The model under review builds one solid part; all positions refer to its coordinate system, in mm. A direction names the side the tool comes from. Coordinates: 2 decimals unless noted, no trailing zeros. Loops run counter-clockwise (first coordinate to the right, second up) from the corner with the lowest first, then second, coordinate; pieces in that order, holes last. Notation, with made-up numbers: (-20.75, 88.25) -> (12.25, 88.25) arc R21 cw to (12.25, 112.25) -> close; hole circle Ø6 at (23, 41.25). An arc over 180 degrees is marked (long way). One line per question, with ' | ' between items. Start each with the question number.
from build123d import *

# Parameters (mm, degrees)
F0_R     = 3
F1_DEPTH = 3.5
F2_W     = 14
F2_H     = 12.5
F3_DEPTH = 0.7
F4_R     = 10
F4_R_2   = 8.4
F5_DEPTH = 20
F6_R     = 10
F6_R_2   = 5
F7_DEPTH = 2


with BuildPart() as f1:
    # F0 (on Top) → F1 (new body)
    with BuildSketch(Plane.XY):
        with BuildLine():
            Line((-7, 37.141428), (-7, 7.141428))
            ThreePointArc((-7, 7.141428), (0, -10), (7, 7.141428))
            Line((7, 7.141428), (7, 37.141428))
            Line((7, 37.141428), (1.936133, 37.141428))
            Line((1.936133, 37.141428), (1.936133, 9.810779))
            ThreePointArc((1.936133, 9.810779), (-0.065184, 9.999788), (-2.063867, 9.784705))
            Line((-2.063867, 9.784705), (-2.063867, 37.141428))
            Line((-2.063867, 37.141428), (-7, 37.141428))
        make_face()
        Circle(F0_R, mode=Mode.SUBTRACT)
    extrude(amount=F1_DEPTH)

    # F2 (on face) → F3 (cut)
    with BuildSketch(Plane.XY.offset(3.5)):
        with Locations((0, 30.891428)):
            Rectangle(F2_W, F2_H)
    extrude(amount=-F3_DEPTH, mode=Mode.SUBTRACT)

    # F4 (on face) → F5 (join)
    with BuildSketch(Plane.XY.offset(3.5)):
        Circle(F4_R)
        Circle(F4_R_2, mode=Mode.SUBTRACT)
    extrude(amount=F5_DEPTH)

    # F6 (on face) → F7 (join)
    with BuildSketch(Plane.XY.offset(23.5)):
        Circle(F6_R)
        Circle(F6_R_2, mode=Mode.SUBTRACT)
    extrude(amount=F7_DEPTH)


solid = f1.part
1) Consider section A-A, the plane y = 29.5. Write out the cut boundary in (x, z), plus the area to 3 significant figures.
2) Machinability: for faces 4 (the face through (0, -4, 3.5)), 5 (the face through (-2.064, 23, 2)), 6 (the face through (-7, 22, 2)), which of the approach directions +Z, -Z, +X, -X, +Y, -Y give a long, thin tool a straight path to every point of the face, cutting with its end or side? Answer none if there is none.
3) Mouldability with a two-part tool opening along Z and no side actions: class faces 1 (the face through (-3, 0, 2)), 2 (the face through (4, 16, 3.5)), 3 (the face through (8.012, 2.523, 13.36)) as +Z half, -Z half, draft (parallel to the pull), parting line (faces both ways), or undercut.
4) Consider section C-C, the plane z = 2. Write out the cut boundary in (x, y).
5) Insertion check: pin 1 Ø5.5 at (x, y) = (4.5, 15.5) entering from +Z; pin 2 Ø3 at (y, z) = (22, 1.5) entering from -X; pin 3 Ø1.8 at (y, z) = (22, 2) entering from +X. Each pin has a flat end and moves straight along its axis. Give the tip position at first contact, or say it passes through.
6) Wall thickness on L1, parallel to Y at x = 0, z = 13; L2, parallel to Y at x = 0, z = 24.85; L3, parallel to Z at x = 3, y = 5.5: over which ranges is each line inside the solid? List them lowest first.
7) Consider section B-B, the plane x = 0. Write out the cut boundary in (y, z), plus the area to 3 significant figures.
Filled sheet:
1) outline: (-7, 0) -> (-2.06, 0) -> (-2.06, 2.8) -> (-7, 2.8) -> close; (1.94, 0) -> (7, 0) -> (7, 2.8) -> (1.94, 2.8) -> close | area: 28.0 mm^2
2) face 4: none | face 5: +Z, -Z, +Y | face 6: +Z, -Z, -X, +Y
3) face 1: draft | face 2: +Z half | face 3: undercut
4) outline: (-7, 7.14) arc R10 ccw (long way) to (7, 7.14) -> (7, 37.14) -> (1.94, 37.14) -> (1.94, 9.81) arc R10 ccw to (-2.06, 9.78) -> (-2.06, 37.14) -> (-7, 37.14) -> close; hole circle Ø6 at (0, 0)
5) pin 1: z = 3.5 | pin 2: x = -7 | pin 3: x = 7
6) L1: -10 to -8.4, 8.4 to 10 | L2: -10 to -5, 5 to 10 | L3: 0 to 3.5, 23.5 to 25.5
7) outline: (-10, 0) -> (-3, 0) -> (-3, 3.5) -> (-8.4, 3.5) -> (-8.4, 23.5) -> (-5, 23.5) -> (-5, 25.5) -> (-10, 25.5) -> close; (3, 0) -> (10, 0) -> (10, 25.5) -> (5, 25.5) -> (5, 23.5) -> (8.4, 23.5) -> (8.4, 3.5) -> (3, 3.5) -> close | area: 133 mm^2
